The model under review builds one solid part; all positions refer to its coordinate system, in mm. Give positions to 0.01 mm unless a question says otherwise; leave off trailing zeros. Order: outer loops, then holes, each group sorted by start corner. A loop starts at its lowest first (then second) coordinate and runs counter-clockwise, first axis right, second up. Notation, with made-up numbers: (23.5, 49) - (27.5, 49) arc R17 ccw to (27.5, 54) - close; hole circle Ø4 at (87.5, 42.5). An arc over 180 degrees is marked (long way). Write item = value, one per line. Start each with the question number.
1. For P1, Ø2, axis at x = 19.475, z = 19.975, coming from the +Y side; P2, Ø1, axis at x = 16.5, z = 17, coming from the -Y side, all flat-tipped, find the tip position at first contact; note any pin that passes through.
2. We need section C-C, the plane y = 2.85. Give the boundary of the cut face in (x, z) (3 decimals), and give its area (3 significant figures).
3. We need section D-D, the plane x = 20. Give the boundary of the cut face in (y, z), and give its area (3 significant figures).
4. Wall thickness on probe 1 along X at (y, z) = (3.35, 20); probe 2 along Z at (x, y) = (-19.5, 1.7); probe 3 along X at (y, z) = (0.7, 10): over which ranges is each line inside the solid? List them lowest first.
5. We need section B-B, the plane z = 10. Give the boundary of the cut face in (x, y).
6. We need section A-A, the plane x = 0. Give the boundary of the cut face in (y, z), and give its area (3 significant figures).
7. Mouldability with a two-part tool opening along Z and no side actions: class faces 1 (the cylindrical face through (-20.155, 1.726, 21.615)), 2 (the cylindrical face through (0.75, 0.68, 11.8)), 3 (the flat face through (0, 2, 25.75)), 4 (the flat face through (0, 2, -4.25)) as pulls with the +Z half, pulls with the -Z half, needs draft (parallel to the pull), parting line crosses it, or undercut.
from build123d import *

# Parameters (mm, degrees)
SKETCH1_W                                      = 50.5
SKETCH1_H                                      = 51.5
SKETCH1_R                                      = 1.775
BOSS_EXTRUDE1_DEPTH                            = 3.5
CSK_FOR_M3_5_FLAT_HEAD_MACHINE_SCREW1_AT_COUNT = 2
CSK_FOR_M3_5_FLAT_HEAD_MACHINE_SCREW1_AT_PITCH = 20


with BuildPart() as part:
    # Sketch1 → Boss-Extrude1 (new body)
    with BuildSketch(Plane(origin=(0, 0, 0), x_dir=(1, 0, 0), z_dir=(0, 1, 0))):
        Rectangle(SKETCH1_W, SKETCH1_H)
        with Locations(Location((-19.475, 19.975, 0), (0, 0, 270))):
            Circle(SKETCH1_R, mode=Mode.SUBTRACT)
        with Locations(Location((19.475, 19.975, 0), (0, 0, 270))):
            Circle(SKETCH1_R, mode=Mode.SUBTRACT)
        with Locations(Location((19.475, -19.975, 0), (0, 0, 270))):
            Circle(SKETCH1_R, mode=Mode.SUBTRACT)
        with Locations(Location((-19.475, -19.975, 0), (0, 0, 270))):
            Circle(SKETCH1_R, mode=Mode.SUBTRACT)
    extrude(amount=BOSS_EXTRUDE1_DEPTH)

    # Sketch4 → CSK for M3.5 Flat Head Machine Screw1 (revolve, cut)
    with BuildSketch(Plane(origin=(0, 3.5, -10), x_dir=(0, 0, 1), z_dir=(1, 0, 0))):
        Polygon((0, 0), (0, 3.5), (1.95, 3.5), (1.95, 2.15), (4.1, 0), align=None)
    csk_for_m3_5_flat_head_machine_screw1 = revolve(axis=Axis((0, 9.85, -10), (0, -1, 0)), mode=Mode.SUBTRACT)

    # CSK for M3.5 Flat Head Machine Screw1 at: CSK for M3.5 Flat Head Machine Screw1 ×2
    with Locations(*[(0, 0, i * CSK_FOR_M3_5_FLAT_HEAD_MACHINE_SCREW1_AT_PITCH) for i in range(1, CSK_FOR_M3_5_FLAT_HEAD_MACHINE_SCREW1_AT_COUNT)]):
        add(csk_for_m3_5_flat_head_machine_screw1, mode=Mode.SUBTRACT)

    # Split1
    split(bisect_by=Plane.XY.offset(-4.25), keep=Keep.TOP)


solid = part.part
Model answer:
q1.P1 = through
q1.P2 = 0
q2.outline = (-25.25, -4.25) - (25.25, -4.25) - (25.25, 25.75) - (-25.25, 25.75) - close; hole circle Ø3.55 at (-19.475, 19.975); hole circle Ø6.9 at (0, 10); hole circle Ø3.55 at (19.475, 19.975)
q2.area = 1,460 mm2
q3.outline = (0, -4.25) - (3.5, -4.25) - (3.5, 18.28) - (0, 18.28) - close; (0, 21.67) - (3.5, 21.67) - (3.5, 25.75) - (0, 25.75) - close
q3.area = 93.1 mm2
q4.probe_1 = -25.25 to -21.25, -17.7 to 17.7, 21.25 to 25.25
q4.probe_2 = -4.25 to 18.2, 21.75 to 25.75
q4.probe_3 = -25.25 to -1.95, 1.95 to 25.25
q5.outline = (-25.25, 0) - (-1.95, 0) - (-1.95, 1.35) - (-4.1, 3.5) - (-25.25, 3.5) - close; (1.95, 0) - (25.25, 0) - (25.25, 3.5) - (4.1, 3.5) - (1.95, 1.35) - close
q6.outline = (0, -4.25) - (3.5, -4.25) - (3.5, 5.9) - (1.35, 8.05) - (0, 8.05) - close; (0, 11.95) - (1.35, 11.95) - (3.5, 14.1) - (3.5, 25.75) - (0, 25.75) - close
q6.area = 86.7 mm2
q7.face_1 = undercut
q7.face_2 = undercut
q7.face_3 = pulls with the +Z half
q7.face_4 = pulls with the -Z half
